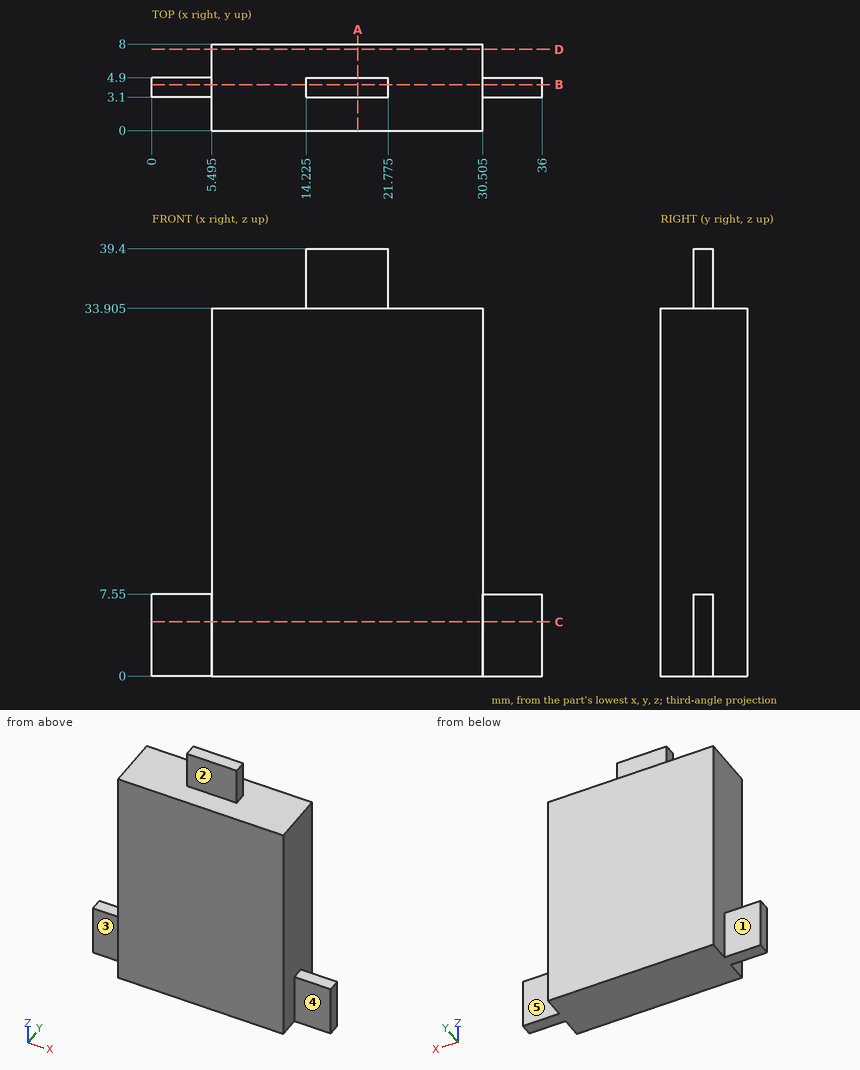
The figure shows three views and two pictorial views of one solid part (mm, origin at its lowest corner). Answer the questions. A direction names the side the tool comes from. Give positions to 0.01 mm unless a question says otherwise; leave off trailing zeros. Write each loop counter-clockwise with the first axis right and the second up, starting at its lowest first coordinate (ties: lowest second). Pieces come first, ordered by that corner, then holes. Notation, with made-up numbers: (-26.5, 59) -> (0.5, 59) arc R22 cw to (0.5, 76) -> close; hole circle Ø11 at (35.5, 3.25). An arc over 180 degrees is marked (long way). Use one line per item in the form item = value.
1) A tool of negligible diameter and unlimited length cuts with its end or side. For the marked faces 1, 2, 3, 4 and 5, from which of +Z, -Z, +X, -X, +Y, -Y can it reach the whole face along a straight path? Write none if from no direction.
Result:
face_1 = +Z, -Z, -X, +Y
face_2 = +Z, +X, -X, -Y
face_3 = +Z, -Z, -X, -Y
face_4 = +Z, -Z, +X, -Y
face_5 = +Z, -Z, +X, +Y
2) Section D-D on y = 7.5 is taken. Write down the section's boundary in (x, z) (3 decimals).
Result:
outline = (5.495, 0) -> (30.505, 0) -> (30.505, 33.905) -> (5.495, 33.905) -> close
3) Section A-A on x = 19 is taken. Write down the section's boundary in (y, z) (3 decimals), plus the area to 3 significant figures.
Result:
outline = (0, 0) -> (8, 0) -> (8, 33.905) -> (4.9, 33.905) -> (4.9, 39.4) -> (3.1, 39.4) -> (3.1, 33.905) -> (0, 33.905) -> close
area = 281 mm²
4) Section C-C on z = 5 is taken. Write down the section's boundary in (x, y) (3 decimals).
Result:
outline = (0, 3.1) -> (5.495, 3.1) -> (5.495, 0) -> (30.505, 0) -> (30.505, 3.1) -> (36, 3.1) -> (36, 4.9) -> (30.505, 4.9) -> (30.505, 8) -> (5.495, 8) -> (5.495, 4.9) -> (0, 4.9) -> close
5) Section B-B on y = 4.25 is taken. Write down the section's boundary in (x, z) (3 decimals), plus the area to 3 significant figures.
Result:
outline = (0, 0) -> (36, 0) -> (36, 7.55) -> (30.505, 7.55) -> (30.505, 33.905) -> (21.775, 33.905) -> (21.775, 39.4) -> (14.225, 39.4) -> (14.225, 33.905) -> (5.495, 33.905) -> (5.495, 7.55) -> (0, 7.55) -> close
area = 972 mm²
6) Each of these flat-tipped pins is pushed along its axis until it touches: P1, Ø1.6, axis at x = 19.5, z = 35.5, coming from the +Y side; P2, Ø4, axis at y = 6, z = 22, coming from the +X side (3 decimals); P3, Ø4, axis at y = 5.5, z = 23.5, coming from the -X side (3 decimals). Where does it stop, or does it pass through?
Result:
P1 = 4.9
P2 = 30.505
P3 = 5.495
7) Straight lines are drawn through the part: probe 1 along X at (y, z) = (1, 26.5) (3 decimals); probe 2 along Z at (x, y) = (20.5, 6.5) (3 decimals); probe 3 along Z at (x, y) = (2, 4). For each, find the intervals that lie inside material, in ascending order.
Result:
probe_1 = 5.495 to 30.505
probe_2 = 0 to 33.905
probe_3 = 0 to 7.55
